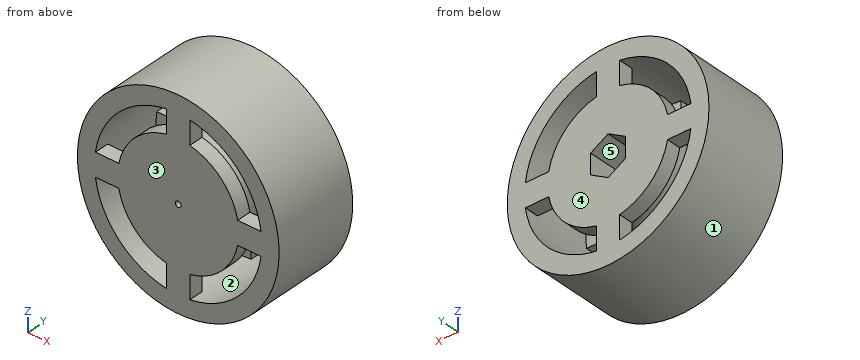
Autodesk Inventor part; units mm, degrees
ref_plane "YZ Plane" through (0, 0, 0) normal (1, 0, 0) x (0, 1, 0)
ref_plane "XZ Plane" through (0, 0, 0) normal (0, 1, 0) x (-1, 0, 0)
ref_plane "XY Plane" through (0, 0, 0) normal (0, 0, 1) x (1, 0, 0)
sketch "Sketch1" plane through (0, 0, 0) normal (0, 1, 0) x (-1, 0, 0)
  circle A0 centre (0, 0) radius 35
  dimension "d0" = 70
extrude "Extrusion1" add sketch "Sketch1" along normal blind 30
sketch "Sketch2" plane through (0, 30, 0) normal (0, 1, 0) x (1, 0, 0)
  circle A0 centre (0, 0) radius 29
  dimension "d3" = 58
extrude "Extrusion2" cut sketch "Sketch2" against normal blind 30
sketch "Sketch3" plane through (0, 30, 0) normal (0, 1, 0) x (1, 0, 0)
  circle A0 centre (0, 0) radius 21
  dimension "d6" = 42
extrude "Extrusion3" add sketch "Sketch3" against normal blind 5
sketch "Sketch4" plane through (0, 25, 0) normal (0, -1, 0) x (1, 0, 0)
  circle A0 centre (0, 0) radius 14
  dimension "d9" = 28
extrude "Extrusion4" add sketch "Sketch4" along normal blind 20
sketch "Sketch5" plane through (0, 5, 0) normal (0, -1, 0) x (1, 0, 0)
  circle A0 centre (0, 0) radius 9
  dimension "d12" = 18
extrude "Extrusion5" cut sketch "Sketch5" against normal blind 20
sketch "Sketch6" plane through (0, 25, 0) normal (0, -1, 0) x (1, 0, 0)
  circle A0 centre (0, 0) radius 9
  dimension "d15" = 18
extrude "Extrusion6" add sketch "Sketch6" along normal blind 12.5
sketch "Sketch8" plane through (0, 12.5, 0) normal (0, -1, 0) x (1, 0, 0)
  circle A0 centre (0, 0) radius 1
  dimension "d26" = 2
extrude "Extrusion8" cut sketch "Sketch8" against normal blind 17.5
sketch "Sketch9" plane through (0, 0, 0) normal (0, -1, 0) x (1, 0, 0)
  circle A0 centre (0, 0) radius 1
  circle A1 centre (0, 0) radius 21
extrude "Extrusion9" add sketch "Sketch9" against normal blind 5
sketch "Sketch10" plane through (0, 30, 0) normal (0, 1, 0) x (1, 0, 0)
  line L0 (17.6248, 0) -> (17.6248, -4)
  line L1 (17.6248, -4) -> (30.6643, -4)
  line L2 (30.6643, -4) -> (30.6643, 4)
  line L3 (30.6643, 4) -> (17.6248, 4)
  line L4 (17.6248, 4) -> (17.6248, 0)
  point P0 (0, 0)
  dimension "d31" = 4
  dimension "d32" = 8
extrude "Extrusion10" add sketch "Sketch10" against normal blind 5
sketch "Sketch11" plane through (0, 30, 0) normal (0, 1, 0) x (1, 0, 0)
  line L0 (0, 30.8076) -> (4, 30.8076)
  line L1 (4, 30.8076) -> (4, 17.4815)
  line L2 (4, 17.4815) -> (-4, 17.4815)
  line L3 (-4, 17.4815) -> (-4, 30.8076)
  line L4 (-4, 30.8076) -> (0, 30.8076)
  point P0 (0, 0)
  dimension "d35" = 4
  dimension "d36" = 8
extrude "Extrusion11" add sketch "Sketch11" against normal blind 5
sketch "Sketch12" plane through (0, 25, 0) normal (0, -1, 0) x (1, 0, 0)
  point P0 (0, 0)
sketch "Sketch13" plane through (0, 30, 0) normal (0, 1, 0) x (1, 0, 0)
  line L0 (0, -17.9114) -> (-4, -17.9114)
  line L1 (-4, -17.9114) -> (-4, -31.0942)
  line L2 (-4, -31.0942) -> (4, -31.0942)
  line L3 (4, -31.0942) -> (4, -17.9114)
  line L4 (4, -17.9114) -> (0, -17.9114)
  point P0 (0, 0)
  dimension "d39" = 4
  dimension "d40" = 8
extrude "Extrusion12" add sketch "Sketch13" against normal blind 5
sketch "Sketch14" plane through (0, 30, 0) normal (0, 1, 0) x (1, 0, 0)
  line L0 (-30.521, 0) -> (-30.521, 4)
  line L1 (-30.521, 4) -> (-18.198, 4)
  line L2 (-18.198, 4) -> (-18.198, -4)
  line L3 (-18.198, -4) -> (-30.521, -4)
  line L4 (-30.521, -4) -> (-30.521, 0)
  point P0 (0, 0)
  dimension "d43" = 4
  dimension "d44" = 8
extrude "Extrusion13" add sketch "Sketch14" against normal blind 5
sketch "Sketch15" plane through (0, 0, 0) normal (0, -1, 0) x (1, 0, 0)
  line L0 (-31.0942, 0) -> (-31.0942, 4)
  line L1 (-31.0942, 4) -> (-17.9114, 4)
  line L2 (-17.9114, 4) -> (-17.9114, -4)
  line L3 (-17.9114, -4) -> (-31.0942, -4)
  line L4 (-31.0942, -4) -> (-31.0942, 0)
  point P0 (0, 0)
  dimension "d47" = 4
  dimension "d48" = 8
extrude "Extrusion14" add sketch "Sketch15" against normal blind 5
sketch "Sketch16" plane through (0, 0, 0) normal (0, -1, 0) x (1, 0, 0)
  line L0 (0, 31.5241) -> (4, 31.5241)
  line L1 (4, 31.5241) -> (4, 16.7651)
  line L2 (4, 16.7651) -> (-4, 16.7651)
  line L3 (-4, 16.7651) -> (-4, 31.5241)
  line L4 (-4, 31.5241) -> (0, 31.5241)
  point P0 (0, 0)
  dimension "d51" = 4
  dimension "d52" = 8
extrude "Extrusion15" add sketch "Sketch16" against normal blind 5
sketch "Sketch17" plane through (0, 0, 0) normal (0, -1, 0) x (1, 0, 0)
  line L0 (31.954, 0) -> (31.954, -4)
  line L1 (31.954, -4) -> (17.6248, -4)
  line L2 (17.6248, -4) -> (17.6248, 4)
  line L3 (17.6248, 4) -> (31.954, 4)
  line L4 (31.954, 4) -> (31.954, 0)
  point P0 (0, 0)
  dimension "d55" = 4
  dimension "d56" = 8
extrude "Extrusion16" add sketch "Sketch17" against normal blind 5
sketch "Sketch18" plane through (0, 0, 0) normal (0, -1, 0) x (1, 0, 0)
  line L0 (0, -31.3808) -> (-4, -31.3808)
  line L1 (-4, -31.3808) -> (-4, -18.3413)
  line L2 (-4, -18.3413) -> (4, -18.3413)
  line L3 (4, -18.3413) -> (4, -31.3808)
  line L4 (4, -31.3808) -> (0, -31.3808)
  point P0 (0, 0)
  dimension "d59" = 4
  dimension "d60" = 8
extrude "Extrusion17" add sketch "Sketch18" against normal blind 5
sketch "Sketch19" plane through (0, 30, 0) normal (0, 1, 0) x (1, 0, 0)
  circle A0 centre (0, 0) radius 1
  line L0 (0, 7) -> (6.0622, 3.5)
  line L1 (6.0622, 3.5) -> (6.0622, -3.5)
  line L2 (6.0622, -3.5) -> (0, -7)
  line L3 (0, -7) -> (-6.0622, -3.5)
  line L4 (-6.0622, -3.5) -> (-6.0622, 3.5)
  line L5 (0, 7) -> (-6.0622, 3.5)
  dimension "d64" = 7
  dimension "d65" = 7
extrude "Extrusion18" cut sketch "Sketch19" against normal blind 16
properties part number "Wheel_2.0"
Input: part model. Units: mm. Frame: model coordinates. Face numbers are marked on the shaded views. A direction names the side the tool comes from. Give positions to 0.01 mm unless a question says otherwise; leave off trailing zeros. Order: outer loops, then holes, each group sorted by start corner. A loop starts at its lowest first (then second) coordinate and runs counter-clockwise, first axis right, second up. Notation, with made-up numbers: M 36.25,-27.5 L 61.25,-27.5 A33 ccw 61.25,2.5 Z; hole C 42.25,-16.5 d3. An arc over 180 degrees is marked long. Return JSON: item names as keys, results as strings.
Item 1: Access query for the marked faces 4 and 5. Directions: +Z, -Z, +X, -X, +Y, -Y. A direction counts if a zero-diameter tool reaches every point of the face in a straight line with its end or side. Return the directions, or none.
Solutions:
{"face 4": "+Z, -Z, +X, -X, +Y", "face 5": "+Y"}
Item 2: Cut plane B-B (y = 23). Return loops of the section in (x, z), then the cut area to 3 significant figures.
Solutions:
{"outline": "C 0,0 d70; C 0,0 d28; hole C 0,0 d58; hole M -6.06,-3.5 L 0,-7 L 6.06,-3.5 L 6.06,3.5 L 0,7 L -6.06,3.5 Z", "area": "1,690 mm^2"}
Item 3: Cut plane D-D (z = -15.5). Return loops of the section in (x, y), then the cut area to 3 significant figures.
Solutions:
{"outline": "M -31.38,0 L -24.51,0 L -24.51,30 L -31.38,30 Z; M -14.17,0 L 14.17,0 L 14.17,5 L -14.17,5 Z; M -14.17,25 L 14.17,25 L 14.17,30 L -14.17,30 Z; M 24.51,0 L 31.38,0 L 31.38,30 L 24.51,30 Z", "area": "696 mm^2"}
Item 4: Pull-direction query (Z, two-part tool) for the marked faces 1, 2 and 3; classes: +Z half, -Z half, draft (parallel to the pull), parting line (faces both ways), or undercut.
Solutions:
{"face 1": "parting line", "face 2": "undercut", "face 3": "draft"}
Item 5: Ray query, probe 1 along Z at (x, y) = (-8, 1.5); probe 2 along Y at (x, z) = (0.5, 22.5); probe 3 along Z at (x, y) = (9, 4.25). Return the intervals inside material, ascending.
Solutions:
{"probe 1": "-34.07 to -27.87, -19.42 to 19.42, 27.87 to 34.07", "probe 2": "0 to 5, 25 to 30", "probe 3": "-33.82 to -27.57, -18.97 to 18.97, 27.57 to 33.82"}
Item 6: Cut plane A-A (z = 0). Return loops of the section in (x, y).
Solutions:
{"outline": "M -35,0 L -1,0 L -1,5 L -9,5 L -9,12.5 L -1,12.5 L -1,14 L -6.06,14 L -6.06,30 L -35,30 Z; M 1,0 L 35,0 L 35,30 L 6.06,30 L 6.06,14 L 1,14 L 1,12.5 L 9,12.5 L 9,5 L 1,5 Z; hole M -29,5 L -14,5 L -14,25 L -29,25 Z; hole M 14,5 L 29,5 L 29,25 L 14,25 Z"}
Item 7: Cut plane C-C (x = -22). Return loops of the section in (y, z).
Solutions:
{"outline": "M 0,-27.22 L 30,-27.22 L 30,-18.89 L 0,-18.89 Z; M 0,-4 L 5,-4 L 5,4 L 0,4 Z; M 0,18.89 L 30,18.89 L 30,27.22 L 0,27.22 Z; M 25,-4 L 30,-4 L 30,4 L 25,4 Z"}
Item 8: First-contact query: P1, Ø2.5, axis at y = 2, z = -23, coming from the -X side; P2, Ø2.5, axis at x = -24, y = 28.5, coming from the -Z side; P3, Ø1.5, axis at x = 13.5, y = 23.5, coming from the +Z side. Flat tips, straight axial feed; report the tip coordinate or a pass-through.
Solutions:
{"P1": "x = -27.42", "P2": "z = -26.6", "P3": "z = 32.6"}
